Read the model definition and answer for the solid it produces. Units are mm, in the model's axes. Face numbers are marked on the shaded views. A direction names the side the tool comes from. Give positions to 0.01 mm unless a question says otherwise; leave off trailing zeros. Loops run counter-clockwise (first coordinate to the right, second up) from the corner with the lowest first, then second, coordinate; pieces in that order, holes last.
(1) Which of the six approach directions +Z, -Z, +X, -X, +Y, -Y give full straight-line access (tool end or side, diameter ignored) to the marked faces 1 and 2?
(2) Each of these flat-tipped pins is pushed along its axis until it touches: P1, Ø1.1, axis at x = 20.5, z = 0.5, coming from the -Y side; P2, Ø6, axis at y = -24.5, z = -10.5, coming from the +X side; P3, Ø0.5, axis at y = -15.5, z = 0.5, coming from the +X side. Where does it stop, or does it pass through?
(3) Straight lines are drawn through the part: probe 1 along X at (y, z) = (-31.5, -4.5); probe 2 along Z at (x, y) = (-27.5, -43); probe 3 along Y at (x, z) = (27.5, -9.5). For each, find the intervals that lie inside material, in ascending order.
(4) Find section C-C, the plane z = -8.25. Write down the section's boundary in (x, y), then the cut area to 3 significant figures.
```python
from build123d import *

# Parameters (mm, degrees)
F1_DEPTH = 1
F3_DEPTH = 15
F4_R     = 1.99999
F5_R     = 10


# Not quite as in the source:
# - a fillet or chamfer is up to 0.001 mm smaller than in the source, because OpenCascade refuses the exact size


with BuildPart() as f1:
    # F0 (on Top) → F1 (new body)
    with BuildSketch(Plane.XY):
        Polygon((-42, -47), (0, -47), (0, 0), (43, 0), (43, 13), (-42, 13), (-42, 0), align=None)
    extrude(amount=F1_DEPTH)

    # F2 (on face) → F3 (join)
    with BuildSketch(Plane(origin=(0, 0, 0), x_dir=(1, 0, 0), z_dir=(0, 0, -1))):
        Polygon((-42, 47), (-42, -13), (-40, -13), (43, -13), (43, -11), (-40, -11), (-40, 47), align=None)
    extrude(amount=F3_DEPTH)

    # F4 (radius 2 in the source; OpenCascade refuses exactly that, so slightly less here)
    f4_edges = [f1.edges().sort_by_distance(p)[0] for p in [
        (-40, -18, -15),
        (1.5, 11, -15),
    ]]
    fillet(f4_edges, radius=F4_R)

    # F5
    f5_edges = [f1.edges().sort_by_distance(p)[0] for p in [
        (0, -47, 0.5),
        (43, 0, 0.5),
    ]]
    fillet(f5_edges, radius=F5_R)


solid = f1.part
```
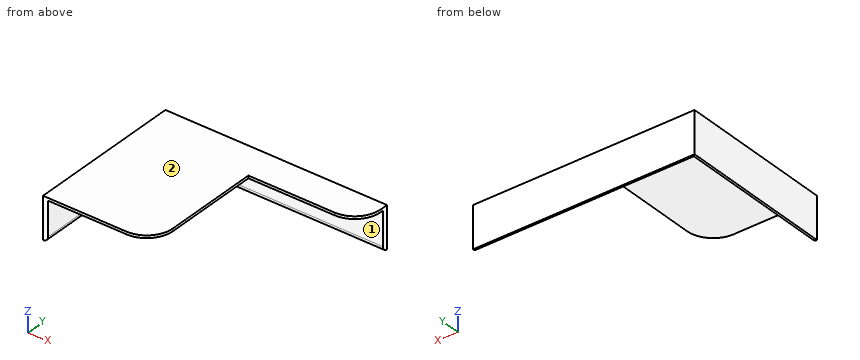
Entries:
1. face 1: -Z, +X, -Y
1. face 2: +Z, +X, -X, +Y, -Y
2. P1: stops at y = 0
2. P2: stops at x = -40
2. P3: stops at x = 0
3. probe 1: x = -42 to -40
3. probe 2: z = 0 to 1
3. probe 3: y = 11 to 13
4. outline: (-42, -47) - (-40, -47) - (-40, 11) - (43, 11) - (43, 13) - (-42, 13) - close
4. area: 286 mm2
